```python
from build123d import *

# Parameters (mm, degrees)
SKETCH035_W     = 46
SKETCH035_H     = 68
PAD010_DEPTH    = 3
FILLET006_R     = 2
SKETCH036_R     = 1.7
POCKET028_DEPTH = 167.305595
POCKET035_DEPTH = 3.001
SKETCH062_R     = 5.15
POCKET043_DEPTH = 167.305595
POCKET044_DEPTH = 3.001


with BuildPart() as part:
    # Sketch035 (on Face1 of CopyMirrored) → Pad010 (new body)
    with BuildSketch(Plane(origin=(0, 0, 45), x_dir=(1, 0, 0), z_dir=(0, 0, -1))):
        with Locations((-21, 0)):
            Rectangle(SKETCH035_W, SKETCH035_H)
    extrude(amount=PAD010_DEPTH)

    # Fillet006
    fillet006_edges = [part.edges().sort_by_distance(p)[0] for p in [
        (-44, -34, 43.5),
        (-44, 34, 43.5),
    ]]
    fillet(fillet006_edges, radius=FILLET006_R)

    # Sketch036 (on Face5 of Fillet006) → Pocket028 (cut, through all)
    with BuildSketch(Plane(origin=(0, 0, 42), x_dir=(1, 0, 0), z_dir=(0, 0, -1))):
        with Locations((-15.2, 15)):
            Circle(SKETCH036_R)
    pocket028 = extrude(amount=-POCKET028_DEPTH, mode=Mode.SUBTRACT)

    # Sketch051 → Pocket035 (cut, through all)
    with BuildSketch(Plane.XY.offset(45)):
        with BuildLine():
            ThreePointArc((-27, 32.5), (-29.5, 30), (-27, 27.5))
            Line((-27, 27.5), (-12, 27.5))
            ThreePointArc((-12, 27.5), (-9.5, 30), (-12, 32.5))
            Line((-27, 32.5), (-12, 32.5))
        make_face()
    extrude(amount=-POCKET035_DEPTH, mode=Mode.SUBTRACT)

    # Sketch062 (on Face5 of Pocket035) → Pocket043 (cut, through all)
    with BuildSketch(Plane(origin=(0, 0, 42), x_dir=(1, 0, 0), z_dir=(0, 0, -1))):
        with Locations((4, 32.5)):
            Circle(SKETCH062_R)
    pocket043 = extrude(amount=-POCKET043_DEPTH, mode=Mode.SUBTRACT)

    # Mirrored006: Pocket043, Pocket028 across XZ
    add(pocket043.mirror(Plane.XZ), mode=Mode.SUBTRACT)
    add(pocket028.mirror(Plane.XZ), mode=Mode.SUBTRACT)

    # Sketch063 (on Face4 of Mirrored006) → Pocket044 (cut, through all)
    with BuildSketch(Plane(origin=(0, 0, 42), x_dir=(1, 0, 0), z_dir=(0, 0, -1))):
        with BuildLine():
            ThreePointArc((-22, 10), (-28, 16), (-34, 10))
            Line((-34, 10), (-34, -10))
            ThreePointArc((-34, -10), (-28, -16), (-22, -10))
            Line((-22, 10), (-22, -10))
        make_face()
    extrude(amount=-POCKET044_DEPTH, mode=Mode.SUBTRACT)


solid = part.part
```
Here's how the part is built. I have some questions about the finished solid (model axes, mm). A direction names the side the tool comes from. Give positions to 0.01 mm unless a question says otherwise; leave off trailing zeros. Write each loop counter-clockwise with the first axis right and the second up, starting at its lowest first coordinate (ties: lowest second). Pieces come first, ordered by that corner, then holes. Notation, with made-up numbers: M 20.5,44 L 38.5,44 A28 cw 38.5,80 Z; hole C -23.5,75 d9. An arc over 180 degrees is marked long. Put each result on its own line as item: value. Start each with the question number.
Item 1: If we section it at D-D, the plane x = -25.5: Write out the boundary of the cut face in (y, z), then the cut area to 3 significant figures.
Item 2: On a 3-axis mill with a long thin cutter (end or side, diameter ignored), from which of +Z, -Z, +X, -X, +Y, -Y can I reach the whole of each face in a straight line? I mean faces 4 (the flat face through (-34, 0, 43)), 5 (the flat face through (-21, 0, 42)). Say none if no direction works.
Item 3: Thinking about a two-plate mould opening in Y: for faces 1 (the cylindrical face through (-16.9, 15.07, 43.48)), 2 (the cylindrical face through (-43.43, 33.4, 43.48)), 3 (the flat face through (-22, -34, 44)), which applies, +Y half, -Y half, draft (parallel to the pull), parting line (faces both ways), or undercut?
Item 4: If we section it at C-C, the plane z = 44.35: Write out the boundary of the cut face in (x, y).
Item 5: I need wall thicknesses on L1, parallel to Y at x = -15.2, z = 42.95; L2, parallel to X at y = -2.5, z = 43.6; L3, parallel to X at y = -15, z = 43.1. Which ranges of each line are inside material? Lowest first, please. Write a range as from..to.
Item 6: If we section it at A-A, the plane y = -1.5: Write out the boundary of the cut face in (x, z), then the cut area to 3 significant figures.
Item 7: If we section it at B-B, the plane x = -18: Write out the boundary of the cut face in (y, z), then the cut area to 3 significant figures.
Values:
1. outline: M -34,42 L -15.45,42 L -15.45,45 L -34,45 Z; M 15.45,42 L 27.5,42 L 27.5,45 L 15.45,45 Z; M 32.5,42 L 34,42 L 34,45 L 32.5,45 Z
1. area: 96.3 mm²
2. face 4: +Z, -Z
2. face 5: -Z, +X, -X, +Y, -Y
3. face 1: undercut
3. face 2: +Y half
3. face 3: -Y half
4. outline: M -44,-32 A2 ccw -42,-34 L -0.93,-34 A5.15 cw 2,-27.75 L 2,27.75 A5.15 cw -0.93,34 L -42,34 A2 ccw -44,32 Z; hole M -34,-10 A6 ccw -22,-10 L -22,10 A6 ccw -34,10 Z; hole M -27,27.5 L -12,27.5 A2.5 ccw -12,32.5 L -27,32.5 A2.5 ccw Z; hole C -15.2,-15 d3.4; hole C -15.2,15 d3.4
5. L1: -34..-16.7, -13.3..13.3, 16.7..27.5, 32.5..34
5. L2: -44..-34, -22..2
5. L3: -44..-31.32, -24.68..-16.9, -13.5..2
6. outline: M -44,42 L -34,42 L -34,45 L -44,45 Z; M -22,42 L 2,42 L 2,45 L -22,45 Z
6. area: 102 mm²
7. outline: M -34,42 L 27.5,42 L 27.5,45 L -34,45 Z; M 32.5,42 L 34,42 L 34,45 L 32.5,45 Z
7. area: 189 mm²
